from build123d import *

# Parameters (mm, degrees)
BOSS_EXTRUDE1_DEPTH = 12.7
HOLE3_D             = 3.175
HOLE3_DEPTH         = 31.75
HOLE3_CSINK_D       = 10.16
HOLE3_CSINK_ANGLE   = 82
HOLE3_TIP           = 0.953866233
HOLE6_D             = 3.175
HOLE6_DEPTH         = 38.1
HOLE6_CSINK_D       = 10.16
HOLE6_CSINK_ANGLE   = 82
HOLE6_TIP           = 0.953866233
HOLE7_D             = 3.175
HOLE7_DEPTH         = 31.75
HOLE7_CSINK_D       = 10.16
HOLE7_CSINK_ANGLE   = 82
HOLE7_TIP           = 0.953866233
HOLE8_D             = 3.175
HOLE8_DEPTH         = 31.75
HOLE8_CSINK_D       = 10.16
HOLE8_CSINK_ANGLE   = 82
HOLE8_TIP           = 0.953866233


with BuildPart() as part:
    # Sketch1 → Boss-Extrude1 (new body)
    with BuildSketch(Plane.XY):
        Polygon((-88.190159952, 0), (-222.052967181, 0), (-222.052967181, -248.25), (-64.977416983, -197.966048293), align=None)
    extrude(amount=-BOSS_EXTRUDE1_DEPTH)

    # Hole3
    with Locations(Plane(origin=(-234.752967181, 1073.364195846, -135.816741379), x_dir=(0, 0, -1), z_dir=(-1, 0, 0))):
        with Locations((-129.466741379, 1300.662770337), (-129.466741379, 1128.612770337), (129.198788767, 1128.612770337), (129.198788767, 1300.662770337)):
            CounterSinkHole(HOLE3_D / 2, HOLE3_CSINK_D / 2, depth=HOLE3_DEPTH, counter_sink_angle=HOLE3_CSINK_ANGLE)
            with Locations((0, 0, -(HOLE3_DEPTH + HOLE3_TIP / 2))):  # 118° drill point
                Cone(0, HOLE3_D / 2, HOLE3_TIP, mode=Mode.SUBTRACT)

    # Hole6
    with Locations(Plane(origin=(181.039434513, 1073.364195846, 0), x_dir=(-0.9271838545667885, -0.3746065934159093, 0), z_dir=(0, 0, 1))):
        with Locations((707.166557203, 1065.270372796), (674.127983646, 944.603090451)):
            CounterSinkHole(HOLE6_D / 2, HOLE6_CSINK_D / 2, depth=HOLE6_DEPTH, counter_sink_angle=HOLE6_CSINK_ANGLE)
            with Locations((0, 0, -(HOLE6_DEPTH + HOLE6_TIP / 2))):  # 118° drill point
                Cone(0, HOLE6_D / 2, HOLE6_TIP, mode=Mode.SUBTRACT)

    # Hole7
    with Locations(Plane(origin=(181.039434513, 12.7, -135.816741379), x_dir=(0, 0, -1), z_dir=(0, 1, 0))):
        with Locations((129.198788767, 384.042401694), (-129.466741379, 384.042401694), (-129.466741379, 304.786761906), (-110.416741379, 409.442401694), (-0.133976306, 409.442401694), (110.148788767, 409.442401694), (129.198788767, 304.786761906)):
            CounterSinkHole(HOLE7_D / 2, HOLE7_CSINK_D / 2, depth=HOLE7_DEPTH, counter_sink_angle=HOLE7_CSINK_ANGLE)
            with Locations((0, 0, -(HOLE7_DEPTH + HOLE7_TIP / 2))):  # 118° drill point
                Cone(0, HOLE7_D / 2, HOLE7_TIP, mode=Mode.SUBTRACT)

    # Hole8
    with Locations(Plane(origin=(531.197640696, -20.449854654, -135.816741379), x_dir=(0, 0, 1), z_dir=(0.3048844921716131, -0.9523893355310409, 0))):
        with Locations((-129.257383629, 761.035393152), (129.466741379, 663.01461615), (129.466741379, 760.835922116), (-129.408220012, 663.214203478)):
            CounterSinkHole(HOLE8_D / 2, HOLE8_CSINK_D / 2, depth=HOLE8_DEPTH, counter_sink_angle=HOLE8_CSINK_ANGLE)
            with Locations((0, 0, -(HOLE8_DEPTH + HOLE8_TIP / 2))):  # 118° drill point
                Cone(0, HOLE8_D / 2, HOLE8_TIP, mode=Mode.SUBTRACT)


solid = part.part
Source: CAD feature listing. Evaluate the final solid. Frame: model axes, mm. Coordinates: 2 decimals unless noted, no trailing zeros. Order: outer loops, then holes, each group sorted by start corner. A loop starts at its lowest first (then second) coordinate and runs counter-clockwise, first axis right, second up.
Item 1: Cut plane C-C (x = -160). Return loops of the section in (y, z).
Output values:
outline: (-228.39, -12.7) - (0, -12.7) - (0, 0) - (-228.39, 0) - close
Item 2: First-contact query: P1, Ø2.5, axis at x = -123.75, z = -6.35, coming from the +Y side; P2, Ø4, axis at x = -90.15, y = -54.99, coming from the -Z side; P3, Ø1, axis at y = -102.5, z = -2, coming from the +X side; P4, Ø2.5, axis at y = -55.25, z = -6.35, coming from the -X side. Flat tips, straight axial feed; report the tip coordinate or a pass-through.
Output values:
P1: stops at y = -19.25
P2: stops at z = -12.7
P3: stops at x = -76.11
P4: stops at x = -202.8
Item 3: Cut plane A-A (z = -10.5). Count the separate pieces of the cut face and the enclosed holes in it, plus the area to 3 significant figures.
Output values:
separate pieces: 1
enclosed holes: 2
area: 32,700 mm2
Item 4: Material intervals for line 1 (X direction, y = -11.5, z = -6.35); line 2 (Y direction, x = -210, z = -6.5); line 3 (X direction, y = -8.75, z = -6.35), sorted ascending.
Output values:
line 1: x = -222.05 to -204.59, -201.42 to -125.33, -122.16 to -86.84
line 2: y = -244.39 to -228.88, -225.72 to -56.83, -53.67 to 0
line 3: x = -222.05 to -204.59, -201.42 to -125.33, -122.16 to -87.16
Item 5: Pull-direction query (Y, two-part tool) for faces 1 (the face through (-222.053, -122, -6)), 2 (the face through (-154, 0, -6)), 3 (the face through (-76.572, -177.799, -3.823)); classes: pulls with the +Y half, pulls with the -Y half, needs draft (parallel to the pull), parting line crosses it, or undercut.
Output values:
face 1: needs draft
face 2: pulls with the +Y half
face 3: undercut
Item 6: Cut plane B-B (y = -79). Return loops of the section in (x, z), plus the area to 3 significant figures.
Output values:
outline: (-222.05, -12.7) - (-78.93, -12.7) - (-78.93, 0) - (-222.05, 0) - close
area: 1,820 mm2
